from build123d import *

# Parameters (mm, degrees)
SKETCH_W        = 40
SKETCH_H        = 38
PAD_DEPTH       = 38
SKETCH001_W     = 38
SKETCH001_H     = 38
POCKET_DEPTH    = 36
SKETCH002_R     = 1.6
POCKET001_DEPTH = 2
SKETCH004_R     = 3
POCKET002_DEPTH = 3
SKETCH005_R     = 1.6
POCKET003_DEPTH = 3
SKETCH006_R     = 2.2
POCKET004_DEPTH = 1.3
SKETCH007_R     = 7.8
POCKET005_DEPTH = 2


with BuildPart() as part:
    # Sketch → Pad (new body)
    with BuildSketch(Plane.XY):
        with Locations((-1, 0)):
            Rectangle(SKETCH_W, SKETCH_H)
    extrude(amount=PAD_DEPTH)

    # Sketch001 (on Face6 of Pad) → Pocket (cut)
    with BuildSketch(Plane.XY.offset(38)):
        Rectangle(SKETCH001_W, SKETCH001_H)
    extrude(amount=-POCKET_DEPTH, mode=Mode.SUBTRACT)

    # Sketch002 (on Face4 of Pocket) → Pocket001 (cut)
    with BuildSketch(Plane.XY.offset(2)):
        with Locations((13.500611, 13.5)):
            Circle(SKETCH002_R)
        with Locations((-13.499389, -13.5)):
            Circle(SKETCH002_R)
        with Locations((13.500611, -13.5)):
            Circle(SKETCH002_R)
        with Locations((-13.499389, 13.5)):
            Circle(SKETCH002_R)
        with Locations((-16.6, 16.6)):
            Circle(SKETCH002_R)
        with Locations((16.6, 16.6)):
            Circle(SKETCH002_R)
        with Locations((16.6, -16.6)):
            Circle(SKETCH002_R)
        with Locations((-16.6, -16.6)):
            Circle(SKETCH002_R)
    extrude(amount=-POCKET001_DEPTH, mode=Mode.SUBTRACT)

    # Sketch004 (on Face5 of Pocket001) → Pocket002 (cut)
    with BuildSketch(Plane.YZ.offset(-19)):
        with Locations((0, 5.624065)):
            Circle(SKETCH004_R)
    extrude(amount=-POCKET002_DEPTH, mode=Mode.SUBTRACT)

    # Sketch005 (on Face5 of Pocket002) → Pocket003 (cut)
    with BuildSketch(Plane.YZ.offset(-19)):
        with Locations((-9, 28)):
            Circle(SKETCH005_R)
        with Locations((9, 28)):
            Circle(SKETCH005_R)
    extrude(amount=-POCKET003_DEPTH, mode=Mode.SUBTRACT)

    # Sketch006 (on Face5 of Pocket003) → Pocket004 (cut)
    with BuildSketch(Plane.YZ.offset(-19)):
        with Locations((-9, 28)):
            Circle(SKETCH006_R)
        with Locations((9, 28)):
            Circle(SKETCH006_R)
    extrude(amount=-POCKET004_DEPTH, mode=Mode.SUBTRACT)

    # Sketch007 (on Face4 of Pocket004) → Pocket005 (cut)
    with BuildSketch(Plane.XY.offset(2)):
        Circle(SKETCH007_R)
    extrude(amount=-POCKET005_DEPTH, mode=Mode.SUBTRACT)


solid = part.part
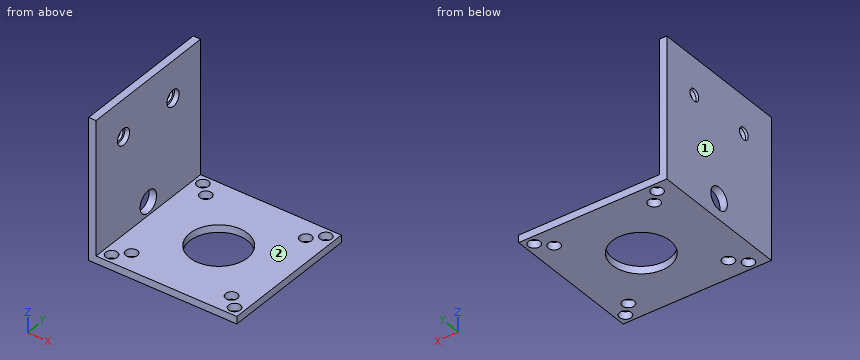
Part model, mm, in its own coordinate system. Face numbers are marked on the shaded views. A direction names the side the tool comes from. Round coordinates to 2 decimals unless told otherwise and drop trailing zeros. Write each loop counter-clockwise with the first axis right and the second up, starting at its lowest first coordinate (ties: lowest second). Pieces come first, ordered by that corner, then holes. Notation, with made-up numbers: M 5.5,-39 L 30.5,-39 A21 ccw 30.5,-11 Z; hole C 50,88.25 d3. An arc over 180 degrees is marked long. Return JSON: item names as keys, results as strings. Group by question number.
(1) Which spindle directions (+Z, -Z, +X, -X, +Y, -Y) get a long thin tool onto all of the face, cutting with end or side? Do the marked faces 1 and 2. Say none if no direction does.
(2) Pin check, flat tips, straight feed: pin 1 Ø1.3 at (y, z) = (-9.5, 27) entering from +X; pin 2 Ø3.5 at (x, y) = (-16.6, 16.6) entering from +Z; pin 3 Ø4 at (y, z) = (3.5, 15.5) entering from +X. Stop position of each tip, or through.
(3) Saw through at C-C on y = -16.6. Write the cut outline in (x, z), then the cut area to 3 significant figures.
(4) Saw through at B-B on x = 16.6. Write the cut outline in (y, z), then the cut area to 3 significant figures.
(5) Saw through at A-A on y = -9. Write the cut outline in (x, z), then the cut area to 3 significant figures.
(6) Drill centre lines: probe 1 along Y at (x, z) = (16.6, 1.05); probe 2 along Z at (x, y) = (-20, 0); probe 3 along Z at (x, y) = (-20.75, -9). Where is each one in solid material? Low to high.
(7) Saw through at D-D on z = 28. Write the cut outline in (x, y).
Returned:
{
 "1": {"face 1": "+Z, -Z, -X, +Y, -Y", "face 2": "+Z, +X, +Y, -Y"},
 "2": {"pin 1": "x = -20.3", "pin 2": "z = 2", "pin 3": "x = -19"},
 "3": {"outline": "M -21,0 L -18.2,0 L -18.2,2 L -19,2 L -19,38 L -21,38 Z; M -15,0 L 15,0 L 15,2 L -15,2 Z; M 18.2,0 L 19,0 L 19,2 L 18.2,2 Z", "area": "139 mm²"},
 "4": {"outline": "M -19,0 L -18.2,0 L -18.2,2 L -19,2 Z; M -15,0 L 15,0 L 15,2 L -15,2 Z; M 18.2,0 L 19,0 L 19,2 L 18.2,2 Z", "area": "63.2 mm²"},
 "5": {"outline": "M -21,0 L 19,0 L 19,2 L -19,2 L -19,25.8 L -20.3,25.8 L -20.3,26.4 L -21,26.4 Z; M -21,29.6 L -20.3,29.6 L -20.3,30.2 L -19,30.2 L -19,38 L -21,38 Z", "area": "144 mm²"},
 "6": {"probe 1": "-19 to -18.2, -15 to 15, 18.2 to 19", "probe 2": "0 to 2.62, 8.62 to 38", "probe 3": "0 to 26.4, 29.6 to 38"},
 "7": {"outline": "M -21,-19 L -19,-19 L -19,-11.2 L -20.3,-11.2 L -20.3,-10.6 L -21,-10.6 Z; M -21,-7.4 L -20.3,-7.4 L -20.3,-6.8 L -19,-6.8 L -19,6.8 L -20.3,6.8 L -20.3,7.4 L -21,7.4 Z; M -21,10.6 L -20.3,10.6 L -20.3,11.2 L -19,11.2 L -19,19 L -21,19 Z"}
}
